from build123d import *

# Parameters (mm, degrees)
SKETCH1_R               = 20
BOSS_EXTRUDE1_DEPTH     = 320
CUT_EXTRUDE1_DEPTH      = 322.247568084
CUT_EXTRUDE1_DEPTH_BACK = 322.247568084
SKETCH2_R               = 4


with BuildPart() as part:
    # Sketch1 → Boss-Extrude1 (new body)
    with BuildSketch(Plane.XY):
        Circle(SKETCH1_R)
    extrude(amount=BOSS_EXTRUDE1_DEPTH)

    # Sketch2 → Cut-Extrude1 (cut, two sides: drawn at the far end of the back side and taken through both)
    with BuildSketch(Plane(origin=(0, 0, 0), x_dir=(0, 0, -1), z_dir=(1, 0, 0)).offset(-CUT_EXTRUDE1_DEPTH_BACK)):
        with Locations(Location((-40, 0, 0), (0, 0, 180))):
            Circle(SKETCH2_R)
        with Locations((-90, 0)):
            Circle(SKETCH2_R)
        with Locations((-310, 0)):
            Circle(SKETCH2_R)
        with Locations((-280, 0)):
            Circle(SKETCH2_R)
    extrude(amount=CUT_EXTRUDE1_DEPTH + CUT_EXTRUDE1_DEPTH_BACK, mode=Mode.SUBTRACT)


solid = part.part
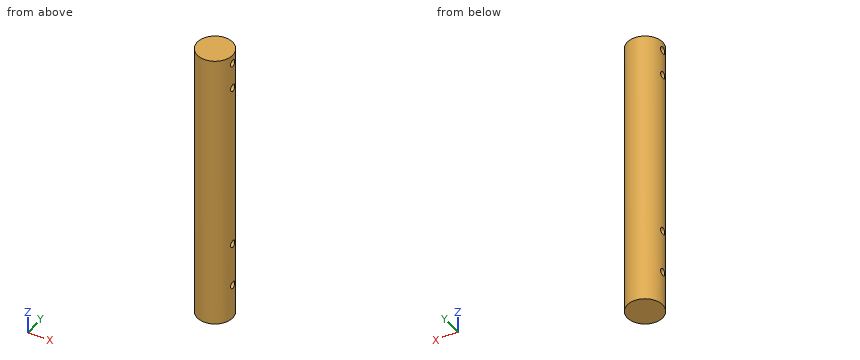
Part model, mm, in its own coordinate system. Coordinates: 2 decimals unless noted, no trailing zeros. Write each loop counter-clockwise with the first axis right and the second up, starting at its lowest first coordinate (ties: lowest second). Pieces come first, ordered by that corner, then holes. Notation, with made-up numbers: (-26, 25.5) - (14, 25.5) arc R17 cw to (14, 43.5) - close; hole circle Ø7 at (-39.5, 87.5). An arc over 180 degrees is marked (long way). Put each result on its own line as item: value.
1. Band-saw the part on C-C (x = 0). Write the cut outline in (y, z).
Final values:
outline: (-20, 0) - (20, 0) - (20, 320) - (-20, 320) - close; hole circle Ø8 at (0, 40); hole circle Ø8 at (0, 90); hole circle Ø8 at (0, 280); hole circle Ø8 at (0, 310)
2. Band-saw the part on D-D (z = 73). Write the cut outline in (x, y).
Final values:
outline: circle Ø40 at (0, 0)
3. Probe line 1 along Y through (x, z) = (-2, 280); line 2 along Y through (x, z) = (-1, 280); line 3 along X through (y, z) = (1, 114.5). List the from-to ranges inside material, lowest first. Write a range as [from, to].
Final values:
line 1: y = [-19.9, -4], [4, 19.9]
line 2: y = [-19.97, -4], [4, 19.97]
line 3: x = [-19.97, 19.97]
4. Band-saw the part on A-A (y = 0). Write the cut outline in (x, z), then the cut area to 3 significant figures.
Final values:
outline: (-20, 0) - (20, 0) - (20, 36) - (-20, 36) - close; (-20, 44) - (20, 44) - (20, 86) - (-20, 86) - close; (-20, 94) - (20, 94) - (20, 276) - (-20, 276) - close; (-20, 284) - (20, 284) - (20, 306) - (-20, 306) - close; (-20, 314) - (20, 314) - (20, 320) - (-20, 320) - close
area: 11,500 mm²
5. Band-saw the part on B-B (x = 12). Write the cut outline in (y, z), then the cut area to 3 significant figures.
Final values:
outline: (-16, 0) - (16, 0) - (16, 320) - (-16, 320) - close; hole circle Ø8 at (0, 40); hole circle Ø8 at (0, 90); hole circle Ø8 at (0, 280); hole circle Ø8 at (0, 310)
area: 10,000 mm²
6. Flat gauge pins, fed straight in: pin 1 Ø12 at (x, z) = (-5.5, 180) entering from +Y; pin 2 Ø2 at (x, z) = (0.5, 78) entering from -Y; pin 3 Ø3 at (y, z) = (8, 222) entering from -X. Where does each tip first touch, or does it go through?
Final values:
pin 1: stops at y = 20
pin 2: stops at y = -20
pin 3: stops at x = -18.91
